Model file for the job. Use its own axes, mm. A direction names the side the tool comes from. Coordinates: 2 decimals unless noted, no trailing zeros. Write each loop counter-clockwise with the first axis right and the second up, starting at its lowest first coordinate (ties: lowest second). Pieces come first, ordered by that corner, then holes. Notation, with made-up numbers: M 42,-3 L 80,-3 A27 cw 80,25 Z; hole C 59.25,82.25 d7. An arc over 180 degrees is marked long. Answer in a Markdown table with one row per item. Add a question column.
```python
from build123d import *

# Parameters (mm, degrees)
SKETCH_2_W                = 28
SKETCH_2_H                = 20.4
EXTRUDE_2_DEPTH           = 7
SKETCH_5_W                = 28
SKETCH_5_H                = 17
EXTRUDE_3_DEPTH           = 18
SKETCH_6_W                = 28
SKETCH_6_H                = 17
EXTRUDE_4_DEPTH           = 18
HOLE_WIZARD_2_D           = 3.4
HOLE_WIZARD_2_CSINK_D     = 6.6
HOLE_WIZARD_2_CSINK_ANGLE = 90
FILLET_1_R                = 10
SKETCH_18_W               = 8
SKETCH_18_H               = 18
EXTRUDE_5_DEPTH           = 12
SKETCH_19_R               = 1.5
CUT_EXTRUDE_6_DEPTH       = 56.673692171
FILLET_2_R                = 2


with BuildPart() as part:
    # 草图2 → 凸台-拉伸2 (new body)
    with BuildSketch(Plane.XY):
        with Locations((14, 10.2)):
            Rectangle(SKETCH_2_W, SKETCH_2_H)
    extrude(amount=EXTRUDE_2_DEPTH)

    # 草图5 → 凸台-拉伸3 (add)
    with BuildSketch(Plane(origin=(0, 20.4, 0), x_dir=(1, 0, 0), z_dir=(0, 1, 0))):
        with Locations((14, -8.5)):
            Rectangle(SKETCH_5_W, SKETCH_5_H)
    extrude(amount=EXTRUDE_3_DEPTH)

    # 草图6 → 凸台-拉伸4 (add)
    with BuildSketch(Plane.XZ):
        with Locations((14, 8.5)):
            Rectangle(SKETCH_6_W, SKETCH_6_H)
    extrude(amount=EXTRUDE_4_DEPTH)

    # 打孔尺寸(%根据十字)槽半沉头木螺钉的类型2 (through all)
    with Locations(Plane(origin=(0, 0, 0), x_dir=(-1, 0, 0), z_dir=(0, 0, -1))):
        with Locations((-22, 17.7), (-6, 17.7), (-6, 2.7), (-22, 2.7)):
            CounterSinkHole(HOLE_WIZARD_2_D / 2, HOLE_WIZARD_2_CSINK_D / 2, counter_sink_angle=HOLE_WIZARD_2_CSINK_ANGLE)

    # 圆角1
    fillet_1_edges = [part.edges().sort_by_distance(p)[0] for p in [
        (14, 38.4, 0),
        (14, -18, 0),
    ]]
    fillet(fillet_1_edges, radius=FILLET_1_R)

    # 草图18 → 凸台-拉伸5 (add)
    with BuildSketch(Plane.XY.offset(17)):
        with Locations((4, 29.4)):
            Rectangle(SKETCH_18_W, SKETCH_18_H)
        with Locations((4, -9)):
            Rectangle(SKETCH_18_W, SKETCH_18_H)
    extrude(amount=EXTRUDE_5_DEPTH)

    # 草图19 → 切除-拉伸6 (cut, through all)
    with BuildSketch(Plane.ZY):
        with Locations((23.5, 29.4)):
            Circle(SKETCH_19_R)
        with Locations((23.5, -9)):
            Circle(SKETCH_19_R)
    extrude(amount=-CUT_EXTRUDE_6_DEPTH, mode=Mode.SUBTRACT)

    # 圆角2
    fillet_2_edges = [part.edges().sort_by_distance(p)[0] for p in [
        (28, 29.4, 17),
        (28, -9, 17),
        (0, 29.4, 29),
        (0, -9, 29),
    ]]
    fillet(fillet_2_edges, radius=FILLET_2_R)


solid = part.part
```
1) Slice it at C-C (z = 11.75). Give the cut face in (x, y).
2) Slice it at A-A (x = 6). Give the cut face in (y, z).
3) Which spindle directions (+Z, -Z, +X, -X, +Y, -Y) get a long thin tool onto all of the face, cutting with end or side? Do faces 1 (the face through (14, 10, 7)), 2 (the face through (22.914, 19.133, 4.338)), 3 (the face through (8, 29.3, 21.6)). Say none if no direction does.
4) Slice it at D-D (x = 22). Give the cut face in (y, z), then the cut area to 3 significant figures.
5) Flat gauge pins, fed straight in: pin 1 Ø3.5 at (y, z) = (29.4, 23.5) entering from -X; pin 2 Ø9.5 at (y, z) = (26.5, 21.5) entering from +X; pin 3 Ø3 at (x, z) = (21, 19.5) entering from -Y; pin 4 Ø2 at (y, z) = (26, 23.5) entering from +X. Where does each tip first touch, or does it go through?
6) Slice it at B-B (y = 22.5). Give the cut face in (x, z), then the cut area to 3 significant figures.
7) Drill centre lines: probe 1 along Y at (x, z) = (3.25, 23.5); probe 2 along X at (y, z) = (17.7, 5.2); probe 3 along Y at (x, z) = (6, 3.2). Where is each one in solid material? Low to high.
8) Two-plate mould, pull along X, no slides. Class faces 4 (the face through (0.57, 29.53, 28.4)), 5 (the face through (14.2, 35.39, 2.85)), 6 (the face through (23.57, 2.05, 4.34)): released by +X, released by -X, zero draft, split by the parting line, or undercut.
Ans:
| question | item | result |
|---|---|---|
| 1 | outline | M 0,-18 L 28,-18 L 28,0 L 0,0 Z; M 0,20.4 L 28,20.4 L 28,38.4 L 0,38.4 Z |
| 2 | outline | M -18,10 A10 ccw -8,0 L -0.6,0 L 1,1.6 L 1,7 L 0,7 L 0,29 L -18,29 Z; M 4.4,1.6 L 6,0 L 14.4,0 L 16,1.6 L 16,7 L 4.4,7 Z; M 19.4,1.6 L 21,0 L 28.4,0 A10 ccw 38.4,10 L 38.4,29 L 20.4,29 L 20.4,7 L 19.4,7 Z; hole C -9,23.5 d3; hole C 29.4,23.5 d3 |
| 3 | face 1 | +Z, +X, -X |
| 3 | face 2 | +Z, -Z |
| 3 | face 3 | +Z, +X, +Y, -Y |
| 4 | outline | M -18,10 A10 ccw -8,0 L -0.6,0 L 1,1.6 L 1,7 L 0,7 L 0,17 L -18,17 Z; M 4.4,1.6 L 6,0 L 14.4,0 L 16,1.6 L 16,7 L 4.4,7 Z; M 19.4,1.6 L 21,0 L 28.4,0 A10 ccw 38.4,10 L 38.4,17 L 20.4,17 L 20.4,7 L 19.4,7 Z |
| 4 | area | 659 mm2 |
| 5 | pin 1 | stops at x = 0 |
| 5 | pin 2 | stops at x = 26.97 |
| 5 | pin 3 | passes through |
| 5 | pin 4 | stops at x = 8 |
| 6 | outline | M 0,0 L 28,0 L 28,15 A2 ccw 26,17 L 8,17 L 8,29 L 2,29 A2 ccw 0,27 Z |
| 6 | area | 570 mm2 |
| 7 | probe 1 | y = -18 to -10.5, -7.5 to 0, 20.4 to 27.9, 30.9 to 38.4 |
| 7 | probe 2 | x = 0 to 4.3, 7.7 to 20.3, 23.7 to 28 |
| 7 | probe 3 | y = -15.33 to 1, 4.4 to 16, 19.4 to 35.73 |
| 8 | face 4 | released by -X |
| 8 | face 5 | zero draft |
| 8 | face 6 | undercut |
